Could you check a few things on this model? Use its own coordinates, in mm. A direction names the side the tool comes from. Give positions to 0.01 mm unless a question says otherwise; leave off trailing zeros. Write each loop counter-clockwise with the first axis right and the second up, starting at its lowest first coordinate (ties: lowest second). Pieces come first, ordered by that corner, then holes. Notation, with made-up numbers: (8, 16) - (40, 16) arc R15 ccw to (40, 41) - close; hole circle Ø5 at (44, 72). An arc over 180 degrees is marked (long way). Answer as a JSON object with one key per item and string values. Group by question number.
```python
from build123d import *

# Parameters (mm, degrees)
BOSS_EXTRUDE1_DEPTH = 88.9
LPATTERN2_COUNT     = 7
LPATTERN2_PITCH     = 25.4
SKETCH4_W           = 18.597058872
SKETCH4_H           = 20.764352928
SKETCH4_W_2         = 25.241981834
SKETCH4_H_2         = 23.038412947
CUT_EXTRUDE1_DEPTH  = 90.473640677


with BuildPart() as part:
    # Sketch1 → Boss-Extrude1 (new, symmetric)
    with BuildSketch(Plane.XY):
        Polygon((-6.096, 7.874), (6.096, 7.874), (3.048, 4.572), (6.35, 1.524), (6.35, 0), (-6.35, 0), (-6.35, 1.524), (-3.048, 4.572), align=None)
    extrude(amount=BOSS_EXTRUDE1_DEPTH, both=True)

    # Sketch2 → Cut-Revolve1 (revolve, cut)
    with BuildSketch(Plane(origin=(0, 0, 0), x_dir=(0, 0, -1), z_dir=(1, 0, 0)), mode=Mode.PRIVATE) as cut_revolve1_sk:
        Polygon((-78.9813, 7.874), (-78.9813, 4.3688), (-77.9272, 4.3688), (-77.9272, 0), (-76.2, 0), (-76.2, 7.874), align=None)
    cut_revolve1 = revolve(cut_revolve1_sk.sketch.rotate(Axis((0, 0, 76.2), (0, 1, 0)), 180), axis=Axis((0, 0, 76.2), (0, 1, 0)), mode=Mode.SUBTRACT)

    # LPattern2: Cut-Revolve1 ×7
    with Locations(*[(0, 0, -i * LPATTERN2_PITCH) for i in range(1, LPATTERN2_COUNT)]):
        add(cut_revolve1, mode=Mode.SUBTRACT)

    # Sketch4 → Cut-Extrude1 (cut, through all)
    with BuildSketch(Plane(origin=(0, 7.874, 0), x_dir=(1, 0, 0), z_dir=(0, 1, 0))):
        with Locations((0, 78.962176464)):
            Rectangle(SKETCH4_W, SKETCH4_H)
        with Locations((0, -80.099206474)):
            Rectangle(SKETCH4_W_2, SKETCH4_H_2)
    extrude(amount=-CUT_EXTRUDE1_DEPTH, mode=Mode.SUBTRACT)


solid = part.part
```
(1) For faces 5 (the flat face through (0, 4.369, -2)), 6 (the cylindrical face through (-0.519, 2.154, -52.447)), 7 (the flat face through (-4.72, 3.03, 0.96)), which set-ups out of +Z, -Z, +X, -X, +Y, -Y let a thin tool reach every point of the face, with its end or its side?
(2) Will these pins go through, and if not, where does the flat tip stop? P1, Ø1.7, axis at x = -1, z = 50.5, coming from the +Y side; P2, Ø3, axis at x = 0, z = 25.4, coming from the -Y side.
(3) I want a section at B-B, the plane y = 6.5. Please give me the cut outline in (x, z).
(4) I want a section at A-A, the plane z = 50.8. Please give me the cut outline in (x, y), and give its area (3 significant figures).
(5) I want a section at C-C, the plane x = 4.5. Please give me the cut outline in (y, z) (3 decimals).
(6) If we mould it in two halves opening along Y, with no side actions, what happens to faces 1 (the flat face through (4.593, 6.246, 0.96)), 2 (the flat face through (2, 0, 1)), 3 (the flat face through (4.676, 3.069, 0.96)), 4 (the cylindrical face through (-0.84, 6.1, -53.45))? For each: +Y half, -Y half, draft (parallel to the pull), parting line (faces both ways), or undercut.
(7) I need wall thicknesses on L1, parallel to Z at x = 0.5, y = 5.5; L2, parallel to Y at x = -1, z = 2.5; L3, parallel to Y at x = -5, z = 36.5. Which ranges of each line are inside material? Lowest first, please.
Entries:
{
 "1": {"face 5": "+Y", "face 6": "+Y, -Y", "face 7": "+Z, -Z, -X"},
 "2": {"P1": "y = 4.37", "P2": "through"},
 "3": {"outline": "(-4.83, -68.58) - (4.83, -68.58) - (4.83, 68.58) - (-4.83, 68.58) - close; hole circle Ø5.56 at (0, -50.8); hole circle Ø5.56 at (0, -25.4); hole circle Ø5.56 at (0, 0); hole circle Ø5.56 at (0, 25.4); hole circle Ø5.56 at (0, 50.8)"},
 "4": {"outline": "(-6.35, 0) - (-1.73, 0) - (-1.73, 4.37) - (-2.78, 4.37) - (-2.78, 7.87) - (-6.1, 7.87) - (-3.05, 4.57) - (-6.35, 1.52) - close; (1.73, 0) - (6.35, 0) - (6.35, 1.52) - (3.05, 4.57) - (6.1, 7.87) - (2.78, 7.87) - (2.78, 4.37) - (1.73, 4.37) - close", "area": "43.6 mm^2"},
 "5": {"outline": "(0, -68.58) - (3.232, -68.58) - (3.232, 68.58) - (0, 68.58) - close; (6.145, -68.58) - (7.874, -68.58) - (7.874, 68.58) - (6.145, 68.58) - close"},
 "6": {"face 1": "undercut", "face 2": "-Y half", "face 3": "undercut", "face 4": "draft"},
 "7": {"L1": "-68.58 to -53.54, -48.06 to -28.14, -22.66 to -2.74, 2.74 to 22.66, 28.14 to 48.06, 53.54 to 68.58", "L2": "0 to 4.37", "L3": "0 to 2.77, 6.69 to 7.87"}
}
